Geometry: final body of the model. Coordinates: model frame, mm. Give positions to 0.01 mm unless a question says otherwise; leave off trailing zeros. Loops run counter-clockwise (first coordinate to the right, second up) from the corner with the lowest first, then second, coordinate; pieces in that order, holes last. Notation, with made-up numbers: (31.25, -27) -> (76.25, -27) arc R34 cw to (76.25, 8) -> close; hole circle Ø8 at (-35, 30). An arc over 180 degrees is marked (long way). One line per question, with ' | ' between items. Start each with the question number.
Item 1: Section C-C on z = -186. Return loops of the section in (x, y).
Item 2: Pin query (flat end, axial travel): P1, Ø3, axis at x = -58, y = 4.5, coming from the -Z side; P2, Ø3, axis at x = -119.5, y = 3, coming from the -Z side; P3, Ø3, axis at y = 3.5, z = -167.5, coming from the +X side. Return the tip coordinate at first contact, or that it passes through.
Item 3: Section B-B on x = -155. Return loops of the section in (y, z).
Item 4: Section A-A on y = 4.5. Return loops of the section in (x, z).
Item 5: Material intervals for line 1 along Z through (x, y) = (-33, 1.5); line 2 along X through (y, z) = (2.25, -211); line 3 along Z through (x, y) = (-165, 2.5), sorted ascending. Write a range as [from, to].
Autodesk Inventor part; units mm, degrees
ref_plane "YZ Plane" through (0, 0, 0) normal (1, 0, 0) x (0, 1, 0)
ref_plane "XZ Plane" through (0, 0, 0) normal (0, 1, 0) x (-1, 0, 0)
ref_plane "XY Plane" through (0, 0, 0) normal (0, 0, 1) x (1, 0, 0)
sketch "Sketch1" plane through (0, 0, 0) normal (0, 1, 0) x (-1, 0, 0)
  point P0 (0, 0)
sketch "Sketch2" plane through (0, 0, 0) normal (0, 1, 0) x (-1, 0, 0)
  line L0 (0, 0) -> (177.8, 0)
  line L1 (177.8, 0) -> (177.8, -203.2)
  line L2 (0, 0) -> (0, -88.9)
  line L3 (177.8, -203.2) -> (107.95, -203.2)
  line L4 (107.95, -203.2) -> (107.95, -88.9)
  line L5 (0, -88.9) -> (107.95, -88.9)
  line L6 (152.1206, -203.2) -> (133.6294, -203.2)
  line L7 (133.6294, -203.2) -> (133.6294, -245.6434)
  line L8 (133.6294, -245.6434) -> (152.1206, -245.6434)
  line L9 (152.1206, -245.6434) -> (152.1206, -203.2)
  dimension "d0" = 203.2
  dimension "d1" = 177.8
  dimension "d2" = 88.9
  dimension "d3" = 69.85
  dimension "d7" = 18.4912
  dimension "d8" = 42.4434
  dimension "d9" = 25.6794
extrude "Extrusion1" add sketch "Sketch2" along normal blind 6.35
properties part number "RSX bottom" material "Aluminum 6061"
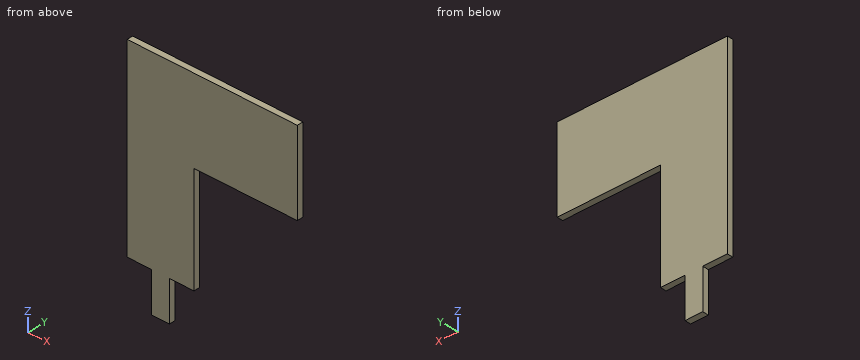
Result sheet:
1) outline: (-177.8, 0) -> (-107.95, 0) -> (-107.95, 6.35) -> (-177.8, 6.35) -> close
2) P1: stops at z = -88.9 | P2: stops at z = -203.2 | P3: stops at x = -107.95
3) outline: (0, -203.2) -> (6.35, -203.2) -> (6.35, 0) -> (0, 0) -> close
4) outline: (-177.8, -203.2) -> (-152.12, -203.2) -> (-152.12, -245.64) -> (-133.63, -245.64) -> (-133.63, -203.2) -> (-107.95, -203.2) -> (-107.95, -88.9) -> (0, -88.9) -> (0, 0) -> (-177.8, 0) -> close
5) line 1: z = [-88.9, 0] | line 2: x = [-152.12, -133.63] | line 3: z = [-203.2, 0]
